Input: part model. Units: mm. Frame: model coordinates. Face numbers are marked on the shaded views. Round coordinates to 2 decimals unless told otherwise and drop trailing zeros. Loops run counter-clockwise (first coordinate to the right, second up) from the corner with the lowest first, then second, coordinate; pieces in that order, holes last.
1) Section A-A, the plane x = -30. Return loops of the section in (y, z), and give its area (3 significant figures).
2) Ray query, line 1 along X through (y, z) = (9.4, 144.5); line 2 along X through (y, z) = (9.95, 160.25); line 3 along X through (y, z) = (10.4, 160.25). Return the intervals inside material, ascending.
3) Section C-C, the plane z = 49. Return loops of the section in (x, y).
4) First-contact query: pin 1 (1.5 mm diameter, centred on x = 19.5, z = 53, fed in from -Y); pin 2 (0.6 mm diameter, centred on x = -7.5, y = 8.5, fed in from -Z); pin 3 (1.5 mm diameter, centred on y = 9.5, z = 139.5, fed in from +X). Flat tips, straight axial feed; report the tip coordinate or a pass-through.
5) Draft query along Y for the marked faces 1 and 2. Return one class per face: pulls with the +Y half, pulls with the -Y half, needs draft (parallel to the pull), parting line crosses it, or undercut.
6) Section B-B, the plane z = 135. Return loops of the section in (x, y).
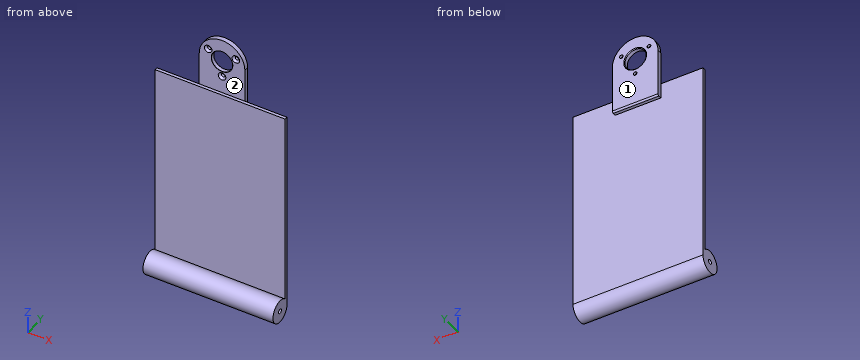
from build123d import *

# Parameters (mm, degrees)
SKETCH1_R           = 1.5
BOSS_EXTRUDE1_DEPTH = 42.8
BOSS_EXTRUDE2_DEPTH = 3
BOSS_EXTRUDE3_DEPTH = 30
CUT_EXTRUDE1_REACH  = 178.227
SKETCH4_R           = 7.000000000000002
SKETCH5_R           = 1.200000000000002
SKETCH5_R_2         = 1.199999999999986
SKETCH5_R_3         = 1.2000000000000053
CUT_EXTRUDE2_DEPTH  = 0.1
CIRPATTERN1_COUNT   = 3


with BuildPart() as part:
    # Sketch1 → Boss-Extrude1 (new, symmetric)
    with BuildSketch(Plane(origin=(0, 0, 0), x_dir=(0, 0, -1), z_dir=(1, 0, 0))):
        with BuildLine():
            Line((-9.2e-16, 7.500000000000001), (-133, 7.499999999999983))
            Line((-133, 7.499999999999983), (-133, 5.499999999999983))
            Line((-133, 5.499999999999983), (-5.099019513592791, 5.499999999999995))
            ThreePointArc((-5.099019513592791, 5.499999999999995), (2.738612787525835, -6.982120021884469), (-9.2e-16, 7.500000000000001))
        make_face()
        Circle(SKETCH1_R, mode=Mode.SUBTRACT)
    extrude(amount=BOSS_EXTRUDE1_DEPTH, both=True)



with BuildPart() as body_2:
    # Sketch2 → Boss-Extrude2 (new body)
    with BuildSketch(Plane(origin=(0, 7.500000000000001, 9.8e-16), x_dir=(1, 0, 0), z_dir=(0, 1, 1.3e-16))):
        with BuildLine():
            Line((15.000000000000007, -155), (15.000000000000007, -133))
            Line((15.000000000000007, -133), (-15.000000000000007, -133))
            Line((-15.000000000000007, -133), (-15.000000000000007, -155))
            ThreePointArc((-15.000000000000007, -155), (-2.76e-15, -170), (15.000000000000007, -155))
        make_face()
    extrude(amount=BOSS_EXTRUDE2_DEPTH)


with BuildPart() as part_1:
    add(part.part)

    add(body_2.part)  # Boss-Extrude3 merges body 2
    # Sketch3 → Boss-Extrude3 (add)
    with BuildSketch(Plane(origin=(15.000000000000007, 0, 0), x_dir=(0, 0, -1), z_dir=(1, 0, 0))):
        with BuildLine():
            Line((-133, 10.499999999999984), (-133, 7.499999999999983))
            Line((-133, 7.499999999999983), (-123.00000000000001, 7.500000000000002))
            Line((-123.00000000000001, 7.500000000000002), (-123.00000000000001, 9.499999999999975))
            ThreePointArc((-123.00000000000001, 9.499999999999975), (-123.29289321881346, 10.207106781186528), (-124.00000000000001, 10.499999999999984))
            Line((-124.00000000000001, 10.499999999999984), (-133, 10.499999999999984))
        make_face()
    extrude(amount=-BOSS_EXTRUDE3_DEPTH)

    # Sketch4 → Cut-Extrude1 (cut, up to next)
    with BuildSketch(Plane(origin=(0, 10.499999999999984, 0), x_dir=(1, 0, 0), z_dir=(0, 1, 0)), mode=Mode.PRIVATE) as cut_extrude1_sk1:
        with Locations(Location((0, -155, 0), (0, 0, 270))):
            Circle(SKETCH4_R)
    cut_extrude1_tool1 = extrude(cut_extrude1_sk1.sketch, amount=-CUT_EXTRUDE1_REACH, mode=Mode.PRIVATE) & part_1.part
    add(cut_extrude1_tool1.solids().sort_by_distance((0, 10.5, 155))[0], mode=Mode.SUBTRACT)

    # Sketch5 → Cut-Extrude2 (cut)
    with BuildSketch(Plane(origin=(0, 10.499999999999984, 0), x_dir=(1, 0, 0), z_dir=(0, 1, 0))):
        with Locations(Location((0, -144.5, 0), (0, 0, 270))):
            Circle(SKETCH5_R)
        with Locations(Location((9.093266739737038, -160.24999999999977, 0), (0, 0, 270))):
            Circle(SKETCH5_R_2)
        with Locations(Location((-9.093266739736205, -160.25000000000017, 0), (0, 0, 270))):
            Circle(SKETCH5_R_3)
    extrude(amount=-CUT_EXTRUDE2_DEPTH, mode=Mode.SUBTRACT)

    # Sketch6 → Cut-Revolve1 (revolve, cut)
    with BuildSketch(Plane(origin=(0, 0, 0), x_dir=(0, 0, -1), z_dir=(1, 0, 0)), mode=Mode.PRIVATE) as cut_revolve1_sk:
        Polygon((-144.5, 7.499999999999982), (-142, 7.4999999999999805), (-143.29999999999998, 8.799999999999951), (-143.29999999999998, 9.799999999999965), (-143.29999999999998, 10.499999999999984), (-144.5, 10.499999999999984), align=None)
    cut_revolve1 = revolve(cut_revolve1_sk.sketch.rotate(Axis((0, 10.499999999999984, 144.5), (0, -1, 0)), 180), axis=Axis((0, 10.499999999999984, 144.5), (0, -1, 0)), mode=Mode.SUBTRACT)

    # CirPattern1: Cut-Revolve1 ×3 about axis
    cirpattern1_axis = Axis((-4.63e-15, 0, 155), (0, 1, 0))
    for i in range(1, CIRPATTERN1_COUNT):
        add(cut_revolve1.rotate(cirpattern1_axis, i * 360 / CIRPATTERN1_COUNT), mode=Mode.SUBTRACT)

    # Sketch7 → Cut-Revolve2 (revolve, cut)
    with BuildSketch(Plane(origin=(0, 0, 0), x_dir=(0, 0, -1), z_dir=(1, 0, 0))):
        Polygon((-148, 7.499999999999981), (-147.9, 7.499999999999981), (-148, 7.599999999999977), align=None)
        Polygon((-148, 10.499999999999984), (-147.5, 10.499999999999984), (-148, 9.99999999999998), (-155, 9.99999999999998), (-155, 10.499999999999984), align=None)
    revolve(axis=Axis((0, 7.4999999999999805, 155), (0, 1, 0)), mode=Mode.SUBTRACT)


solid = part_1.part
Final values:
1. outline: (5.5, 5.1) arc R7.5 ccw (long way) to (7.5, 0) - (7.5, 133) - (5.5, 133) - close; hole circle Ø3 at (0, 0)
1. area: 429 mm2
2. line 1: x = -15 to -1.2, 1.2 to 15
2. line 2: x = -14.05 to -10.29, -7.89 to -4.63, 4.63 to 7.89, 10.29 to 14.05
2. line 3: x = -14.05 to -10.29, -7.89 to -5.22, 5.22 to 7.89, 10.29 to 14.05
3. outline: (-42.8, 5.5) - (42.8, 5.5) - (42.8, 7.5) - (-42.8, 7.5) - close
4. pin 1: stops at y = 5.5
4. pin 2: stops at z = 123
4. pin 3: stops at x = 15
5. face 1: pulls with the +Y half
5. face 2: pulls with the -Y half
6. outline: (-15, 7.5) - (15, 7.5) - (15, 10.5) - (-15, 10.5) - close
